from build123d import *

# Parameters (mm, degrees)
SKETCH1_W                  = 152.4
SKETCH1_H                  = 2.38125
BOSS_EXTRUDE1_DEPTH        = 76.2
F_31_0_12_DIAMETER_HOLE4_D = 3.048
SKETCH25_W                 = 73.533
SKETCH25_H                 = 8.89
BOSS_EXTRUDE2_DEPTH        = 2.38125
SKETCH26_W                 = 7.1755
SKETCH26_H                 = 3.175
CUT_EXTRUDE3_DEPTH         = 3.38125
F_31_0_12_DIAMETER_HOLE6_D = 3.048
SKETCH32_W                 = 73.533
SKETCH32_H                 = 6.35
BOSS_EXTRUDE3_DEPTH        = 2.38125
SKETCH31_R                 = 1.27
CUT_EXTRUDE4_DEPTH         = 3.38125


with BuildPart() as part:
    # Sketch1 → Boss-Extrude1 (new body)
    with BuildSketch(Plane.XY):
        with Locations((76.2, 1.190625)):
            Rectangle(SKETCH1_W, SKETCH1_H)
    extrude(amount=BOSS_EXTRUDE1_DEPTH)

    # #31 (0.12) Diameter Hole4 (through all)
    with Locations(Plane(origin=(0, 2.38125, 0), x_dir=(1, 0, 0), z_dir=(0, 1, 0))):
        with Locations((49.448559218, -3.690103872), (21.508561504, -3.690103872), (6.268559218, -54.490103872)):
            Hole(F_31_0_12_DIAMETER_HOLE4_D / 2)

    # Sketch25 → Boss-Extrude2 (add)
    with BuildSketch(Plane(origin=(0, 2.38125, 0), x_dir=(1, 0, 0), z_dir=(0, 1, 0))):
        with Locations((81.135059218, 4.445)):
            Rectangle(SKETCH25_W, SKETCH25_H)
        with Locations((81.135059218, -80.645)):
            Rectangle(SKETCH25_W, SKETCH25_H)
    extrude(amount=-BOSS_EXTRUDE2_DEPTH)

    # Sketch26 → Cut-Extrude3 (cut, through all)
    with BuildSketch(Plane(origin=(0, 2.38125, 0), x_dir=(1, 0, 0), z_dir=(0, 1, 0))):
        with Locations((70.816309218, 4.445)):
            Rectangle(SKETCH26_W, SKETCH26_H)
        with Locations((98.819809218, 4.445)):
            Rectangle(SKETCH26_W, SKETCH26_H)
        with Locations((98.819809218, -80.645)):
            Rectangle(SKETCH26_W, SKETCH26_H)
        with Locations((70.816309218, -80.645)):
            Rectangle(SKETCH26_W, SKETCH26_H)
    extrude(amount=-CUT_EXTRUDE3_DEPTH, mode=Mode.SUBTRACT)

    # #31 (0.12) Diameter Hole6 (through all)
    with Locations(Plane(origin=(0, 2.38125, 0), x_dir=(1, 0, 0), z_dir=(0, 1, 0))):
        with Locations((84.818059218, 4.445), (112.821559218, 4.445), (112.821559218, -80.645), (84.818059218, -80.645)):
            Hole(F_31_0_12_DIAMETER_HOLE6_D / 2)

    # Sketch32 → Boss-Extrude3 (add)
    with BuildSketch(Plane.XZ):
        with Locations((81.135059218, 88.265)):
            Rectangle(SKETCH32_W, SKETCH32_H)
        with Locations((81.135059218, -12.065)):
            Rectangle(SKETCH32_W, SKETCH32_H)
    extrude(amount=-BOSS_EXTRUDE3_DEPTH)

    # Sketch31 → Cut-Extrude4 (cut, through all)
    with BuildSketch(Plane(origin=(0, 0, 0), x_dir=(-1, 0, 0), z_dir=(0, -1, 0))):
        with Locations((-148.59, -43.421592432)):
            Circle(SKETCH31_R)
        with Locations((-148.59, -53.581592432)):
            Circle(SKETCH31_R)
    extrude(amount=-CUT_EXTRUDE4_DEPTH, mode=Mode.SUBTRACT)


solid = part.part
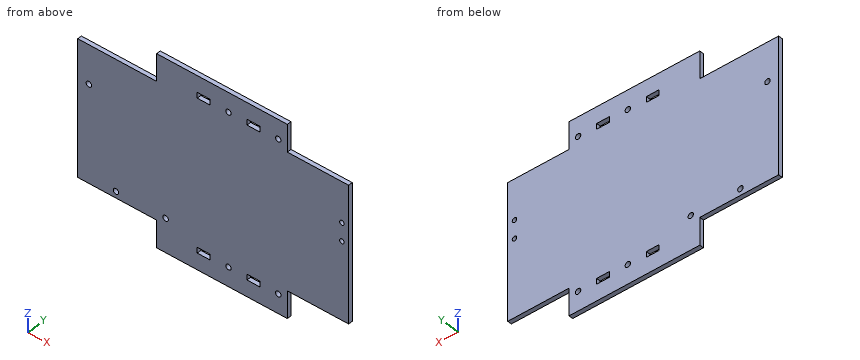
Here's how the part is built. I have some questions about the finished solid (model axes, mm). Coordinates: 2 decimals unless noted, no trailing zeros. Write each loop counter-clockwise with the first axis right and the second up, starting at its lowest first coordinate (ties: lowest second). Pieces come first, ordered by that corner, then holes. Notation, with made-up numbers: (84.5, 81.25) - (137.5, 81.25) arc R25 cw to (137.5, 113.25) - close; hole circle Ø1 at (65, 51). An arc over 180 degrees is marked (long way). Use one line per item in the form item = value.
1) Suppose I cut it at A-A, the plane x = 99. Write out the boundary of the cut face in (y, z), plus the area to 3 significant figures.
Solved:
outline = (0, -15.24) - (2.38, -15.24) - (2.38, -6.03) - (0, -6.03) - close; (0, -2.86) - (2.38, -2.86) - (2.38, 79.06) - (0, 79.06) - close; (0, 82.23) - (2.38, 82.23) - (2.38, 91.44) - (0, 91.44) - close
area = 239 mm2
2) I'm going to push flat-ended pins straight in: P1, Ø1.2, axis at x = 16, y = 0.5, coming from the +Z side; P2, Ø1.2, axis at y = 1.5, z = -4.5, coming from the -X side; P3, Ø0.7, axis at y = 1, z = -4, coming from the +X side. Where does each tip first touch, or does it pass through?
Solved:
P1 = 76.2
P2 = 44.37
P3 = 117.9
3) I need wall thicknesses on line 1 (Z direction, x = 69.5, y = 1.65); line 2 (X direction, y = 0.35, z = 81); line 3 (Z direction, x = 148.59, y = 1.3). Which ranges of each line are inside material? Lowest first, please.
Solved:
line_1 = -15.24 to -6.03, -2.86 to 79.06, 82.23 to 91.44
line_2 = 44.37 to 67.23, 74.4 to 83.34, 86.3 to 95.23, 102.41 to 111.34, 114.3 to 117.9
line_3 = 0 to 42.15, 44.69 to 52.31, 54.85 to 76.2
4) Suppose I cut it at B-B, the plane y = 1.9. Give the number of separate pieces and of enclosed holes in the cut face, plus the area to 3 significant figures.
Solved:
separate_pieces = 1
enclosed_holes = 13
area = 13,700 mm2
5) Suppose I cut it at C-C, the plane x = 17.5. Write out the boundary of the cut face in (y, z), plus the area to 3 significant figures.
Solved:
outline = (0, 0) - (2.38, 0) - (2.38, 76.2) - (0, 76.2) - close
area = 181 mm2
